Study the drawing (mm; zero at the part's minimum x, y, z) and answer. A direction names the side the tool comes from. Give positions to 0.01 mm unless a question says otherwise; leave off trailing zeros. Write each loop counter-clockwise with the first axis right and the second up, starting at its lowest first coordinate (ties: lowest second). Pieces come first, ordered by that corner, then holes. Notation, with made-up numbers: M 59,3.25 L 110,3.25 A31 cw 110,30.25 Z; hole C 76.25,19.25 d11. An arc over 180 degrees is marked long. Use a Markdown table: item, result. Add a question column.
Item 1: A cutting plane is placed at A-A on y = 31. Determine the outline of the cut face in (x, z), then the cut area to 3 significant figures.
Item 2: A cutting plane is placed at D-D on z = 23. Determine the outline of the cut face in (x, y), then the cut area to 3 significant figures.
Item 3: Consider probe 1 along X at (y, z) = (40.25, 10); probe 2 along Y at (x, z) = (42, 37.5); probe 3 along X at (y, z) = (25, 20). Determine where each line is inside the solid, lowest interval first. Write a range as [from, to].
Item 4: Given P1, Ø3, axis at x = 8, z = 10, coming from the -Y side, flat-ended and moving along its own axis, determine where the tip first touches the part or whether it passes through.
Item 5: For the marked faces 4 and 5, determine the directions among +Z, -Z, +X, -X, +Y, -Y from which every point of the face is accessible in a straight line to the end or side of a thin tool.
Item 6: A cutting plane is placed at C-C on x = 20. Determine the outline of the cut face in (y, z).
Item 7: A cutting plane is placed at B-B on z = 10. Count the separate pieces of the cut face and the enclosed holes in it, then the cut area to 3 significant figures.
Item 8: The mould has two halves that part along Y. Classify the marked faces 1, 2 and 3: pulls with the +Y half, pulls with the -Y half, needs draft (parallel to the pull), parting line crosses it, or undercut.
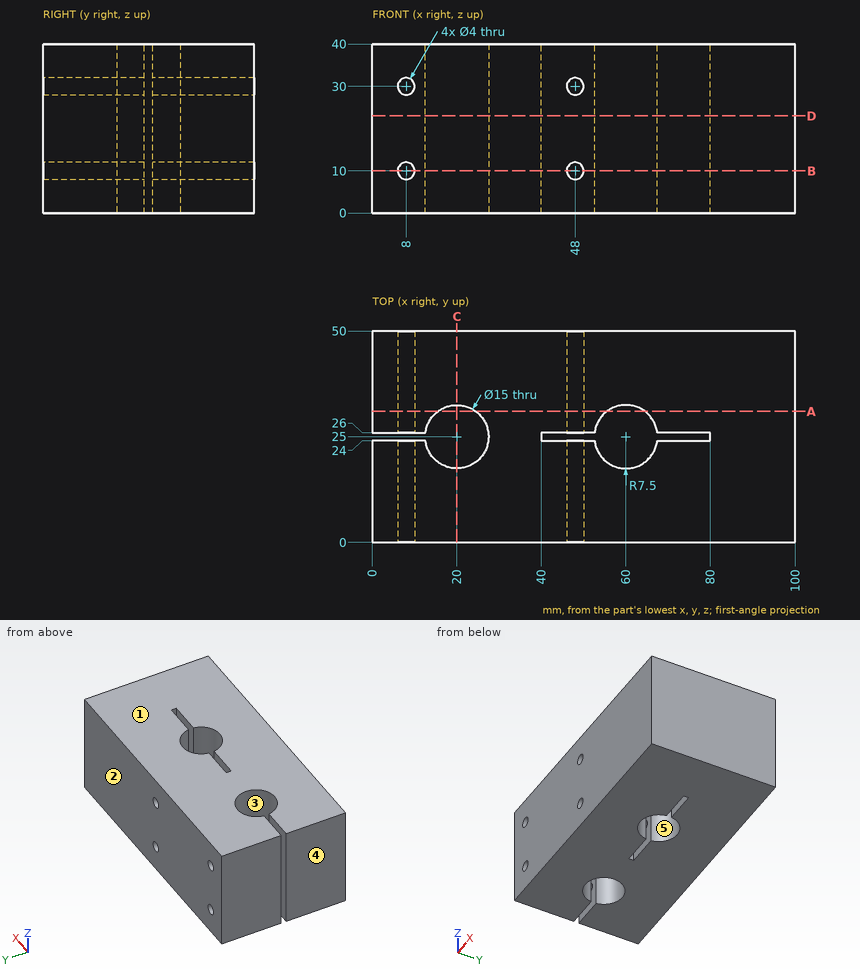
Filled in:
| question | item | result |
|---|---|---|
| 1 | outline | M 0,0 L 15.5,0 L 15.5,40 L 0,40 Z; M 24.5,0 L 55.5,0 L 55.5,40 L 24.5,40 Z; M 64.5,0 L 100,0 L 100,40 L 64.5,40 Z; hole C 8,10 d4; hole C 8,30 d4; hole C 48,10 d4; hole C 48,30 d4 |
| 1 | area | 3,230 mm² |
| 2 | outline | M 0,0 L 100,0 L 100,50 L 0,50 L 0,26 L 12.57,26 A7.5 cw long 12.57,24 L 0,24 Z; hole M 40,24 L 52.57,24 A7.5 ccw 67.43,24 L 80,24 L 80,26 L 67.43,26 A7.5 ccw 52.57,26 L 40,26 Z |
| 2 | area | 4,570 mm² |
| 3 | probe 1 | [0, 6], [10, 46], [50, 100] |
| 3 | probe 2 | [0, 24], [26, 50] |
| 3 | probe 3 | [27.5, 40], [80, 100] |
| 4 | P1 | through |
| 5 | face 4 | +Z, -Z, -X, +Y, -Y |
| 5 | face 5 | +Z, -Z |
| 6 | outline | M 0,0 L 17.5,0 L 17.5,40 L 0,40 Z; M 32.5,0 L 50,0 L 50,40 L 32.5,40 Z |
| 7 | separate pieces | 4 |
| 7 | enclosed holes | 0 |
| 7 | area | 4,190 mm² |
| 8 | face 1 | needs draft |
| 8 | face 2 | pulls with the +Y half |
| 8 | face 3 | undercut |
